from build123d import *

# Parameters (mm, degrees)
SKETCH1_R           = 2.7
SKETCH1_R_2         = 3.56
BOSS_EXTRUDE1_DEPTH = 3.175
CHAMFER1_SIZE       = 3
CHAMFER2_SIZE       = 3


with BuildPart() as part:
    # Sketch1 → Boss-Extrude1 (new body)
    with BuildSketch(Plane(origin=(0, 0, 0), x_dir=(1, 0, 0), z_dir=(0, 1, 0))):
        Polygon((0, 0), (40, 0), (40, -17.5), (57.4, -17.5), (57.4, 37.5), (40, 37.5), (40, 20), (0, 20), align=None)
        with Locations((29, 10)):
            Circle(SKETCH1_R, mode=Mode.SUBTRACT)
        with Locations((9, 10)):
            Circle(SKETCH1_R_2, mode=Mode.SUBTRACT)
        with Locations((48.7, 31.5)):
            Circle(SKETCH1_R, mode=Mode.SUBTRACT)
        with Locations((48.7, -11.5)):
            Circle(SKETCH1_R, mode=Mode.SUBTRACT)
        with Locations((49, 10)):
            Circle(SKETCH1_R, mode=Mode.SUBTRACT)
    extrude(amount=BOSS_EXTRUDE1_DEPTH)

    # Chamfer1
    chamfer1_edges = [part.edges().sort_by_distance(p)[0] for p in [
        (0, 1.5875, -20),
        (40, 1.5875, -37.5),
        (57.4, 1.5875, -37.5),
        (57.4, 1.5875, 17.5),
        (40, 1.5875, 17.5),
        (0, 1.5875, 0),
    ]]
    chamfer(chamfer1_edges, length=CHAMFER1_SIZE)

    # Chamfer2
    chamfer2_edges = [part.edges().sort_by_distance(p)[0] for p in [
        (40, 1.5875, -20),
        (40, 1.5875, 0),
    ]]
    chamfer(chamfer2_edges, length=CHAMFER2_SIZE)


solid = part.part
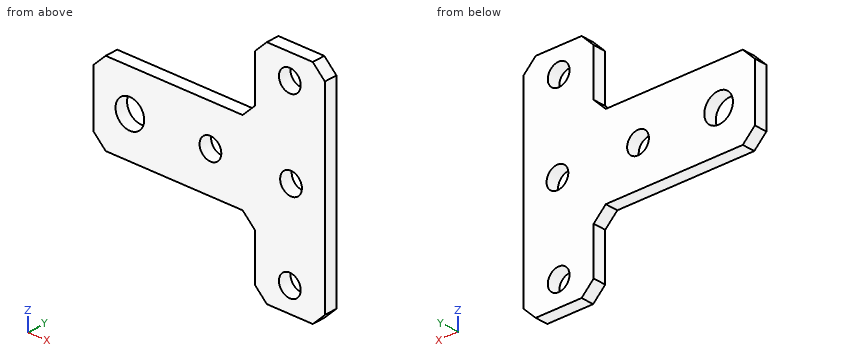
Here's how the part is built. I have some questions about the finished solid (model axes, mm). Give positions to 0.01 mm unless a question says otherwise; leave off trailing zeros. Order: outer loops, then holes, each group sorted by start corner. A loop starts at its lowest first (then second) coordinate and runs counter-clockwise, first axis right, second up. Notation, with made-up numbers: M -26,12 L 28,12 A11 ccw 28,28 Z; hole C -33,61.25 d5. An arc over 180 degrees is marked long. Answer as a JSON object with one key per item and string values. Group by question number.
1) I'm going to push flat-ended pins straight in: pin 1 Ø4.5 at (x, z) = (48.7, -31.5) entering from -Y; pin 2 Ø1.6 at (y, z) = (1, -30) entering from -X. Where does each tip first touch, or does it pass through?
2) Suppose I cut it at C-C, the plane y = 1.7. Write out the boundary of the cut face in (x, z), plus the area to 3 significant figures.
3) Suppose I cut it at A-A, the plane z = -31.5. Write out the boundary of the cut face in (x, y) (3 decimals).
4) Suppose I cut it at B-B, the plane x = 9. Write out the boundary of the cut face in (y, z) (3 decimals).
5) Please list where these lines run through material, in increasing order: L1, parallel to X at y = 1.75, z = -10; L2, parallel to Z at x = 9, y = 1.3; L3, parallel to Z at x = 49, y = 1.65. Write a range as [from, to].
6) Suppose I cut it at D-D, the plane z = -10. Write out the boundary of the cut face in (x, y) (3 decimals).
Results found:
{
 "1": {"pin 1": "through", "pin 2": "x = 40"},
 "2": {"outline": "M 0,-17 L 3,-20 L 37,-20 L 40,-23 L 40,-34.5 L 43,-37.5 L 54.4,-37.5 L 57.4,-34.5 L 57.4,14.5 L 54.4,17.5 L 43,17.5 L 40,14.5 L 40,3 L 37,0 L 3,0 L 0,-3 Z; hole C 9,-10 d7.12; hole C 29,-10 d5.4; hole C 48.7,-31.5 d5.4; hole C 48.7,11.5 d5.4; hole C 49,-10 d5.4", "area": "1,610 mm²"},
 "3": {"outline": "M 40,0 L 46,0 L 46,3.175 L 40,3.175 Z; M 51.4,0 L 57.4,0 L 57.4,3.175 L 51.4,3.175 Z"},
 "4": {"outline": "M 0,-20 L 3.175,-20 L 3.175,-13.56 L 0,-13.56 Z; M 0,-6.44 L 3.175,-6.44 L 3.175,0 L 0,0 Z"},
 "5": {"L1": "[0, 5.44], [12.56, 26.3], [31.7, 46.3], [51.7, 57.4]", "L2": "[-20, -13.56], [-6.44, 0]", "L3": "[-37.5, -34.18], [-28.82, -12.7], [-7.3, 8.82], [14.18, 17.5]"},
 "6": {"outline": "M 0,0 L 5.44,0 L 5.44,3.175 L 0,3.175 Z; M 12.56,0 L 26.3,0 L 26.3,3.175 L 12.56,3.175 Z; M 31.7,0 L 46.3,0 L 46.3,3.175 L 31.7,3.175 Z; M 51.7,0 L 57.4,0 L 57.4,3.175 L 51.7,3.175 Z"}
}
